Build history of the part. All positions in model axes, mm. A direction names the side the tool comes from. Coordinates: 2 decimals unless noted, no trailing zeros. Write each loop counter-clockwise with the first axis right and the second up, starting at its lowest first coordinate (ties: lowest second). Pieces come first, ordered by that corner, then holes. Notation, with made-up numbers: (-12, 41) -> (8, 41) arc R18 cw to (8, 49) -> close; hole circle Ø3 at (88.5, -32.75). An arc over 180 degrees is marked (long way). Write each question's results on one line, items separated by ' | '. Start each with the question number.
Q1. Tool access for faces 5 (the face through (-56.18, 7.85, 646)), 6 (the face through (1, 0, 603)): list every direction of +Z, -Z, +X, -X, +Y, -Y with a clear straight run to the whole face (end or side of a thin tool).
Q2. Drop flat-ended pins along their axis: pin 1 Ø8 at (y, z) = (-15.5, 609.5) entering from +X; pin 2 Ø6 at (y, z) = (-7.5, 628) entering from +X. Give the stop position or say it passes through.
Q3. Saw through at C-C on y = 0. Count the separate pieces of the cut face and the enclosed holes in it, and give its area (3 significant figures).
Q4. Two-plate mould, pull along Y, no slides. Class faces 1 (the face through (63.735, 0.412, 649.76)), 2 (the face through (33.82, -7.85, 607)), 3 (the face through (1, 0, 650)), 4 (the face through (-58.487, 0.594, 649.014)): released by +Y, released by -Y, zero draft, split by the parting line, or undercut.
Q5. Saw through at B-B on x = 37. Give the cut face in (y, z).
Q6. Drill centre lines: line 1 (X direction, y = 0, z = 622); line 2 (Y direction, x = 45, z = 648.5); line 3 (X direction, y = -0.5, z = 626.5). Where is each one in solid material? Low to high.
Q7. Saw through at D-D on z = 616.5. Give the cut face in (x, y).
Q8. Saw through at A-A on z = 626.5. Give the cut face in (x, y).
from build123d import *

# Parameters (mm, degrees)
BOSS_EXTRUDE1_START = 650
SKETCH1_R           = 13.5
BOSS_EXTRUDE1_DEPTH = 47
CUT_EXTRUDE2_START  = -2
SKETCH4_R           = 15
SKETCH4_R_2         = 13.5
CUT_EXTRUDE2_DEPTH  = 2
SKETCH5_R           = 4
CUT_EXTRUDE3_DEPTH  = 40
CUT_EXTRUDE4_START  = -4
SKETCH6_R           = 15
SKETCH6_R_2         = 13.5
CUT_EXTRUDE4_DEPTH  = 2
CHAMFER1_SIZE       = 1.5


with BuildPart() as part:
    # Sketch1 → Boss-Extrude1 (new body)
    with BuildSketch(Plane.XY.offset(BOSS_EXTRUDE1_START)):
        with BuildLine():
            Line((-45, 20), (45, 20))
            ThreePointArc((45, 20), (65, 0), (45, -20))
            Line((45, -20), (-45, -20))
            ThreePointArc((-45, -20), (-65, 0), (-45, 20))
        make_face()
        with Locations((-45, 0)):
            Circle(SKETCH1_R, mode=Mode.SUBTRACT)
        with Locations((45, 0)):
            Circle(SKETCH1_R, mode=Mode.SUBTRACT)
    extrude(amount=-BOSS_EXTRUDE1_DEPTH)

    # Sketch4 → Cut-Extrude2 (cut)
    # profile 1 of 2: a face of its own
    with BuildSketch(Plane.XY.offset(650).offset(CUT_EXTRUDE2_START)):
        with Locations((-45, 0)):
            Circle(SKETCH4_R)
        with Locations((-45, 0)):
            Circle(SKETCH4_R_2, mode=Mode.SUBTRACT)
    # profile 2 of 2: a face of its own
    with BuildSketch(Plane.XY.offset(650).offset(CUT_EXTRUDE2_START)):
        with Locations((45, 0)):
            Circle(SKETCH4_R)
        with Locations((45, 0)):
            Circle(SKETCH4_R_2, mode=Mode.SUBTRACT)
    extrude(amount=-CUT_EXTRUDE2_DEPTH, mode=Mode.SUBTRACT)

    # Sketch5 → Cut-Extrude3 (cut)
    with BuildSketch(Plane(origin=(0, 20, 0), x_dir=(1, 0, 0), z_dir=(0, 1, 0))):
        with Locations(Location((0, -626.5, 0), (0, 0, 270))):
            Circle(SKETCH5_R)
    extrude(amount=-CUT_EXTRUDE3_DEPTH, mode=Mode.SUBTRACT)

    # Sketch6 → Cut-Extrude4 (cut)
    # profile 1 of 2: a face of its own
    with BuildSketch(Plane(origin=(0, 0, 603), x_dir=(-1, 0, 0), z_dir=(0, 0, -1)).offset(CUT_EXTRUDE4_START)):
        with Locations(Location((-45, 0, 0), (0, 0, 180))):
            Circle(SKETCH6_R)
        with Locations(Location((-45, 0, 0), (0, 0, 180))):
            Circle(SKETCH6_R_2, mode=Mode.SUBTRACT)
    # profile 2 of 2: a face of its own
    with BuildSketch(Plane(origin=(0, 0, 603), x_dir=(-1, 0, 0), z_dir=(0, 0, -1)).offset(CUT_EXTRUDE4_START)):
        with Locations(Location((45, 0, 0), (0, 0, 180))):
            Circle(SKETCH6_R)
        with Locations(Location((45, 0, 0), (0, 0, 180))):
            Circle(SKETCH6_R_2, mode=Mode.SUBTRACT)
    extrude(amount=CUT_EXTRUDE4_DEPTH, mode=Mode.SUBTRACT)

    # Chamfer1
    chamfer1_edges = [part.edges().sort_by_distance(p)[0] for p in [
        (65, 0, 603),
        (0, 20, 603),
        (-65, 0, 603),
        (0, 20, 650),
        (65, 0, 650),
        (0, -20, 650),
        (-65, 0, 650),
        (0, -20, 603),
    ]]
    chamfer(chamfer1_edges, length=CHAMFER1_SIZE)


solid = part.part
Returned:
1) face 5: none | face 6: -Z, +X, -X, +Y, -Y
2) pin 1: stops at x = 61.36 | pin 2: stops at x = 64.49
3) separate pieces: 3 | enclosed holes: 1 | area: 3,490 mm2
4) face 1: split by the parting line | face 2: undercut | face 3: zero draft | face 4: undercut
5) outline: (-20, 604.5) -> (-18.5, 603) -> (-10.87, 603) -> (-10.87, 605) -> (-12.69, 605) -> (-12.69, 607) -> (-10.87, 607) -> (-10.87, 646) -> (-12.69, 646) -> (-12.69, 648) -> (-10.87, 648) -> (-10.87, 650) -> (-18.5, 650) -> (-20, 648.5) -> close; (10.87, 603) -> (18.5, 603) -> (20, 604.5) -> (20, 648.5) -> (18.5, 650) -> (10.87, 650) -> (10.87, 648) -> (12.69, 648) -> (12.69, 646) -> (10.87, 646) -> (10.87, 607) -> (12.69, 607) -> (12.69, 605) -> (10.87, 605) -> close
6) line 1: x = -65 to -58.5, -31.5 to 31.5, 58.5 to 65 | line 2: y = -20 to -13.5, 13.5 to 20 | line 3: x = -64.99 to -58.49, -31.51 to -4, 4 to 31.51, 58.49 to 64.99
7) outline: (-45, -20) -> (45, -20) arc R20 ccw to (45, 20) -> (-45, 20) arc R20 ccw to start; hole circle Ø27 at (-45, 0); hole circle Ø27 at (45, 0)
8) outline: (-45, -20) -> (-4, -20) -> (-4, 20) -> (-45, 20) arc R20 ccw to start; (4, -20) -> (45, -20) arc R20 ccw to (45, 20) -> (4, 20) -> close; hole circle Ø27 at (-45, 0); hole circle Ø27 at (45, 0)
